Input: part model. Units: mm. Frame: model coordinates. Give positions to 0.01 mm unless a question says otherwise; leave off trailing zeros. Order: outer loops, then holes, each group sorted by start corner. A loop starts at its lowest first (then second) coordinate and runs counter-clockwise, first axis right, second up. Notation, with made-up numbers: (40, -24) - (81, -24) arc R23 ccw to (81, 7) - close; hole circle Ø3 at (64.5, 70.25). An arc over 180 degrees is marked (long way). Answer in a Markdown table with one row per item. Add a question column.
1. Contact query for a flat-ended pin moving along its axis: pin 1 (2.5 mm diameter, centred on x = 0, y = 0, fed in from -Z). Output: stop coordinate, or through.
2. Mould query, pull axis X, two halves, no side actions, for faces 1 (the face through (3, 0, 0)), 2 (the face through (-1.5, 2.6, 0)), 3 (the face through (-0.24, 3.15, -1.25)), 4 (the face through (2, 0, 0)). Classes: released by +X, released by -X, zero draft, split by the parting line, or undercut.
3. Section query A-A on z = -0.2. Return loops of the section in (x, y).
4. Ray query, line 1 (X direction, y = 0, z = -0.4); line 2 (Y direction, x = -1.6, z = -0.2); line 3 (Y direction, x = -1.65, z = 0.05). Return the intervals inside material, ascending. Write a range as [from, to].
Autodesk Inventor part; units mm, degrees
ref_plane "YZ Plane" through (0, 0, 0) normal (1, 0, 0) x (0, 1, 0)
ref_plane "XZ Plane" through (0, 0, 0) normal (0, 1, 0) x (-1, 0, 0)
ref_plane "XY Plane" through (0, 0, 0) normal (0, 0, 1) x (1, 0, 0)
sketch "Sketch1" plane through (0, 0, 0) normal (0, 0, 1) x (1, 0, 0)
  line L0 (0, 3.4641) -> (3, 1.7321)
  line L1 (3, 1.7321) -> (3, -1.7321)
  line L2 (3, -1.7321) -> (0, -3.4641)
  line L3 (0, -3.4641) -> (-3, -1.7321)
  line L4 (-3, -1.7321) -> (-3, 1.7321)
  line L5 (-3, 1.7321) -> (0, 3.4641)
  circle A0 centre (0, 0) radius 2 construction
  dimension "Diameter" = 4
  dimension "Width_Across_Flats" = 6
extrude "Extrusion1" add sketch "Sketch1" along normal mid plane 2.5
sketch "Sketch2" plane through (0, 0, 0) normal (0, 1, 0) x (-1, 0, 0)
  line L0 (-3, 1.25) -> (-3, -1.25) construction
  line L1 (0, 0) -> (0, 4.375)
  line L2 (-3, 1.25) -> (-5, 1.25)
  line L3 (-5, 1.25) -> (-5, 0.0953)
  line L4 (-5, 0.0953) -> (-3, 1.25)
  dimension "Chamfer_Angle" = 30
  dimension "Chamfer_Size" = 2
revolve "Revolution1" cut sketch "Sketch2" angle 360 about axis through (0, 0, 0) along (0, 0, 1)
sketch "Sketch3" plane through (0, 0, -1.25) normal (0, 0, -1) x (-1, 0, 0)
  line L0 (3, -1.7321) -> (0, -3.4641) construction
  circle A0 centre (0, 0) radius 3
extrude "Extrusion2" add sketch "Sketch3" along normal blind 0.25
hole "Hole1" at (0, 0, 1.25) direction (0, 0, -1) diameter 4 end through all
thread "Thread1"
chamfer "Chamfer1" distance 0.25 angle 45 2 edges at (0, 2, 1.25) (0, 2, -1.5)
equation "\"Width_Across_Flats\" = 1.5 * Diameter"
equation "\"Thickness\" = 0.625 * Diameter"
equation "\"Chamfer_Size\" = 0.5 * Diameter"
equation "\"Hole_Diameter\" = Diameter"
properties part number "Hex Jam Nut with Washer Face"
Answer:
| question | item | result |
|---|---|---|
| 1 | pin 1 | passes through |
| 2 | face 1 | released by +X |
| 2 | face 2 | released by -X |
| 2 | face 3 | zero draft |
| 2 | face 4 | undercut |
| 3 | outline | (-3, -1.73) - (0, -3.46) - (3, -1.73) - (3, 1.73) - (0, 3.46) - (-3, 1.73) - close; hole circle Ø4 at (0, 0) |
| 4 | line 1 | x = [-3, -2], [2, 3] |
| 4 | line 2 | y = [-2.54, -1.2], [1.2, 2.54] |
| 4 | line 3 | y = [-2.51, -1.13], [1.13, 2.51] |
